Can you work these out from the model? Positions are in its coordinate system, mm. Face numbers are marked on the shaded views. Round coordinates to 2 decimals unless told otherwise and drop trailing zeros. Order: outer loops, then holes, each group sorted by start corner. A loop starts at its lowest first (then second) coordinate and runs counter-clockwise, first axis right, second up. Notation, with made-up numbers: (62, 64) -> (71, 64) arc R22 ccw to (71, 72) -> close; hole circle Ø8 at (7, -29). An arc over 180 degrees is marked (long way). Use a Markdown table: item, result. Add a question column.
Q1. I'm going to push flat-ended pins straight in: pin 1 Ø1.5 at (x, y) = (0.5, -1) entering from +Z; pin 2 Ø6 at (x, z) = (-2, -4) entering from +Y. Where does each tip first touch, or does it pass through?
Q2. I need wall thicknesses on line 1 along Z through (x, y) = (-0.25, 3.5); line 2 along Y through (x, z) = (0, 7.75); line 3 along Y through (x, z) = (-0.5, -3.25). Which ranges of each line are inside material? Lowest first, please. Write a range as [from, to].
Q3. We'd pull the mould along Z, two halves only. Please class the marked faces 1, 2 and 3: +Z half, -Z half, draft (parallel to the pull), parting line (faces both ways), or undercut.
Q4. If we section it at C-C on z = 8: List the corners of the cut face in (x, y) for me.
Q5. If we section it at D-D on y = 2: List the corners of the cut face in (x, z) for me.
Q6. If we section it at A-A on x = 0: List the corners of the cut face in (y, z) for me, plus the area to 3 significant figures.
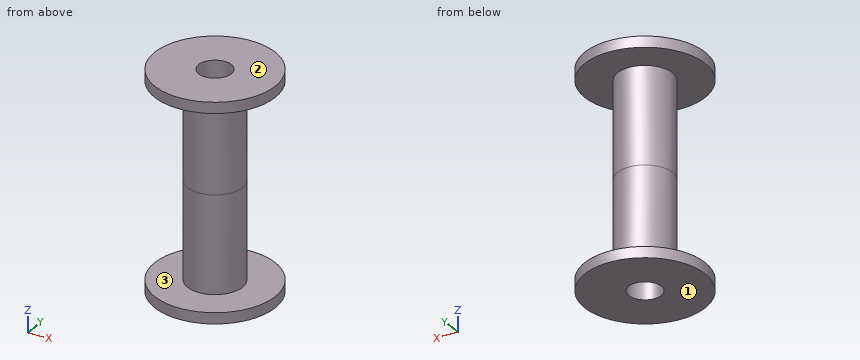
```python
from build123d import *

# Parameters (mm, degrees)
ESQUISSE1_R        = 2.5
ESQUISSE1_R_2      = 1.5
BOSS_EXTRU_1_DEPTH = 9.85
ESQUISSE2_R        = 5.5
ESQUISSE2_R_2      = 2.5
BOSS_EXTRU_2_DEPTH = 1


with BuildPart() as part:
    # Esquisse1 → Boss.-Extru.1 (new body)
    with BuildSketch(Plane.XY):
        Circle(ESQUISSE1_R)
        Circle(ESQUISSE1_R_2, mode=Mode.SUBTRACT)
    boss_extru_1 = extrude(amount=BOSS_EXTRU_1_DEPTH)

    # Esquisse2 → Boss.-Extru.2 (add)
    with BuildSketch(Plane.XY.offset(9.85)):
        Circle(ESQUISSE2_R)
        Circle(ESQUISSE2_R_2, mode=Mode.SUBTRACT)
    boss_extru_2 = extrude(amount=-BOSS_EXTRU_2_DEPTH)

    # Symétrie1: Boss.-Extru.1, Boss.-Extru.2 across plane
    add(boss_extru_1.mirror(Plane.XY))
    add(boss_extru_2.mirror(Plane.XY))


solid = part.part
```
Answer below:
| question | item | result |
|---|---|---|
| 1 | pin 1 | z = 9.85 |
| 1 | pin 2 | y = 2.5 |
| 2 | line 1 | [-9.85, -8.85], [8.85, 9.85] |
| 2 | line 2 | [-2.5, -1.5], [1.5, 2.5] |
| 2 | line 3 | [-2.45, -1.41], [1.41, 2.45] |
| 3 | face 1 | -Z half |
| 3 | face 2 | +Z half |
| 3 | face 3 | undercut |
| 4 | outline | circle Ø5 at (0, 0); hole circle Ø3 at (0, 0) |
| 5 | outline | (-5.12, -9.85) -> (5.12, -9.85) -> (5.12, -8.85) -> (1.5, -8.85) -> (1.5, 8.85) -> (5.12, 8.85) -> (5.12, 9.85) -> (-5.12, 9.85) -> (-5.12, 8.85) -> (-1.5, 8.85) -> (-1.5, -8.85) -> (-5.12, -8.85) -> close |
| 6 | outline | (-5.5, -9.85) -> (-1.5, -9.85) -> (-1.5, 9.85) -> (-5.5, 9.85) -> (-5.5, 8.85) -> (-2.5, 8.85) -> (-2.5, -8.85) -> (-5.5, -8.85) -> close; (1.5, -9.85) -> (5.5, -9.85) -> (5.5, -8.85) -> (2.5, -8.85) -> (2.5, 8.85) -> (5.5, 8.85) -> (5.5, 9.85) -> (1.5, 9.85) -> close |
| 6 | area | 51.4 mm² |
